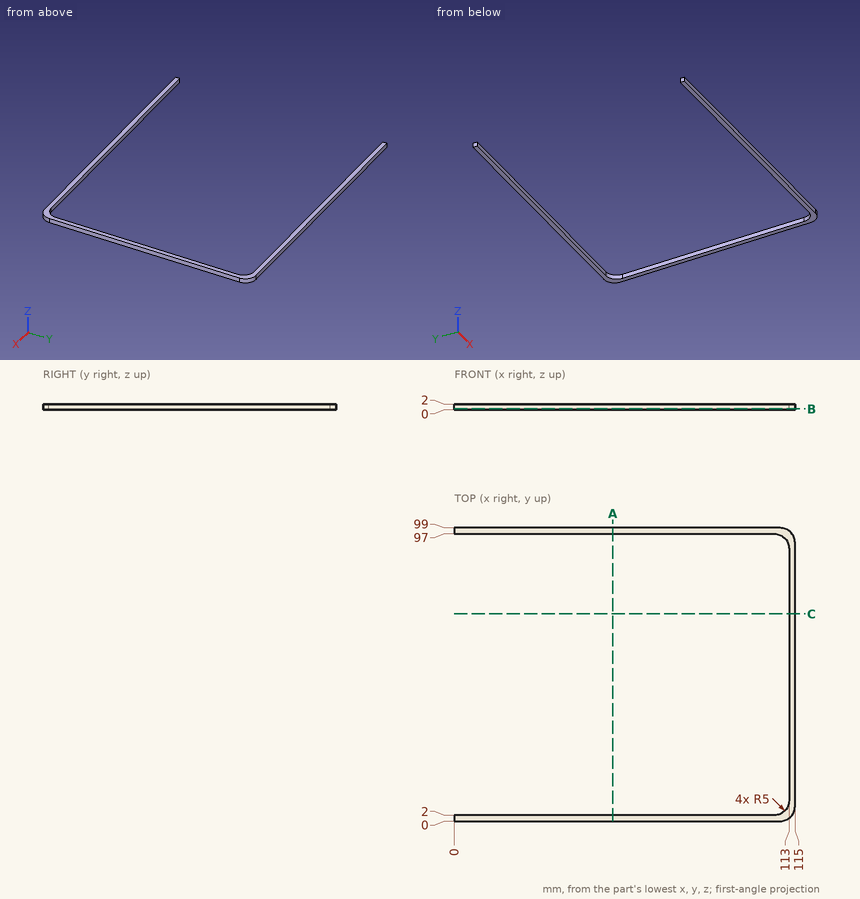
Here's the drawing with two shaded views (mm, measured from the low corner). I have some questions. Coordinates: 2 decimals unless noted, no trailing zeros. Order: outer loops, then holes, each group sorted by start corner. A loop starts at its lowest first (then second) coordinate and runs counter-clockwise, first axis right, second up.
Q1. Suppose I cut it at A-A on x = 53.5. Please give me the cut outline in (y, z).
Q2. Please list where these lines run through material, in increasing order: L1, parallel to Y at x = 60, z = 0.9; L2, parallel to X at y = 11, z = 0.9; L3, parallel to X at y = 94.5, z = 0.8.
Q3. Suppose I cut it at C-C on y = 70. Please give me the cut outline in (x, z), and give its area (3 significant figures).
Q4. Suppose I cut it at B-B on z = 0.35. Please give me the cut outline in (x, y).
Q5. Will this pin go through, and if not, where does the flat tip stop? pin 1 (1 mm diameter, centred on y = 56, z = 1, fed in from -X).
Answer:
1. outline: (0, 0) - (2, 0) - (2, 2) - (0, 2) - close; (97, 0) - (99, 0) - (99, 2) - (97, 2) - close
2. L1: y = 0 to 2, 97 to 99
2. L2: x = 113 to 115
2. L3: x = 112.33 to 114.97
3. outline: (113, 0) - (115, 0) - (115, 2) - (113, 2) - close
3. area: 4.00 mm2
4. outline: (0, 0) - (110, 0) arc R5 ccw to (115, 5) - (115, 94) arc R5 ccw to (110, 99) - (0, 99) - (0, 97) - (108, 97) arc R5 cw to (113, 92) - (113, 7) arc R5 cw to (108, 2) - (0, 2) - close
5. pin 1: stops at x = 113
